Read the model definition and answer for the solid it produces. Units are mm, in the model's axes. Round coordinates to 2 decimals unless told otherwise and drop trailing zeros. Order: outer loops, then holes, each group sorted by start corner. A loop starts at its lowest first (then second) coordinate and runs counter-clockwise, first axis right, second up.
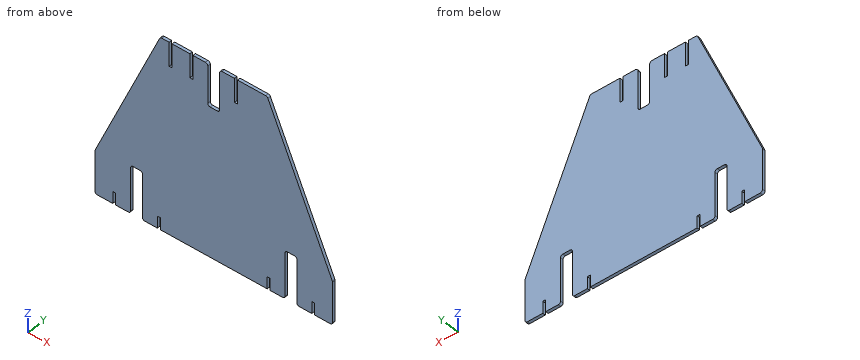
from build123d import *

# Parameters (mm, degrees)
BOSS_EXTRUDE1_DEPTH = 3.0988
FILLET1_R           = 2.54


with BuildPart() as part:
    # Sketch1 → Boss-Extrude1 (new body)
    with BuildSketch(Plane(origin=(0, 0, 0), x_dir=(1, 0, 0), z_dir=(0, 1, 0))):
        Polygon((6.35, -57.15), (-6.35, -57.15), (-6.35, -101.6), (-22.225, -101.6), (-22.225, -76.2), (-25.4, -76.2), (-25.4, -101.6), (-44.45, -101.6), (-44.45, -76.2), (-47.625, -76.2), (-47.625, -101.6), (-57.15, -101.6), (-127, 55.88), (-127, 101.6), (-107.95, 101.6), (-107.95, 88.9), (-104.775, 88.9), (-104.775, 101.6), (-88.9, 101.6), (-88.9, 50.8), (-76.2, 50.8), (-76.2, 101.6), (-60.325, 101.6), (-60.325, 88.9), (-57.15, 88.9), (-57.15, 101.6), (57.15, 101.6), (57.15, 88.9), (60.325, 88.9), (60.325, 101.6), (76.2, 101.6), (76.2, 50.8), (88.9, 50.8), (88.9, 101.6), (104.775, 101.6), (104.775, 88.9), (107.95, 88.9), (107.95, 101.6), (127, 101.6), (127, 55.88), (57.15, -101.6), (25.4, -101.6), (25.4, -76.2), (22.225, -76.2), (22.225, -101.6), (6.35, -101.6), align=None)
    extrude(amount=BOSS_EXTRUDE1_DEPTH)

    # Fillet1
    fillet1_edges = [part.edges().sort_by_distance(p)[0] for p in [
        (88.9, 1.5494, -50.8),
        (88.9, 1.5494, -101.6),
        (127, 1.5494, -101.6),
        (127, 1.5494, -55.88),
        (57.15, 1.5494, 101.6),
        (6.35, 1.5494, 101.6),
        (6.35, 1.5494, 57.15),
        (-6.35, 1.5494, 57.15),
        (-6.35, 1.5494, 101.6),
        (-57.15, 1.5494, 101.6),
        (-127, 1.5494, -55.88),
        (-127, 1.5494, -101.6),
        (-88.9, 1.5494, -101.6),
        (-88.9, 1.5494, -50.8),
        (-76.2, 1.5494, -50.8),
        (-76.2, 1.5494, -101.6),
        (76.2, 1.5494, -101.6),
        (76.2, 1.5494, -50.8),
    ]]
    fillet(fillet1_edges, radius=FILLET1_R)


solid = part.part
Q1. A cutting plane is placed at B-B, the plane x = 82. Give the vertices of the cut face in (y, z).
Outcome:
outline: (0, -50.8) - (3.1, -50.8) - (3.1, 45.57) - (0, 45.57) - close
Q2. A cutting plane is placed at A-A, the plane z = -71. Give the vertices of the cut face in (x, y).
Outcome:
outline: (-127, 0) - (-88.9, 0) - (-88.9, 3.1) - (-127, 3.1) - close; (-76.2, 0) - (76.2, 0) - (76.2, 3.1) - (-76.2, 3.1) - close; (88.9, 0) - (127, 0) - (127, 3.1) - (88.9, 3.1) - close
Q3. A cutting plane is placed at C-C, the plane z = 22. Give the vertices of the cut face in (x, y).
Outcome:
outline: (-92.46, 0) - (92.46, 0) - (92.46, 3.1) - (-92.46, 3.1) - close
Q4. Flat-ended cylindrical pins translate along their axes: pin 1 (1.5 mm diameter, centred on x = -24, y = 2, fed in from +Z); pin 2 (1.5 mm diameter, centred on x = -81.5, y = 1, fed in from -Z); pin 3 (0.9 mm diameter, centred on x = 58.5, y = 1, fed in from -Z); pin 4 (1.5 mm diameter, centred on x = -15, z = -65.5, fed in from -Y). Find the tip coordinate at first contact, or state that the pin passes through.
Outcome:
pin 1: stops at z = 76.2
pin 2: stops at z = -50.8
pin 3: stops at z = -88.9
pin 4: stops at y = 0
Q5. Straight lines are drawn through the part: probe 1 along X at (y, z) = (1, -67); probe 2 along X at (y, z) = (1.2, 70); probe 3 along Z at (x, y) = (-106, 1.4). For each, find the intervals that lie inside material, in ascending order.
Outcome:
probe 1: x = -127 to -88.9, -76.2 to 76.2, 88.9 to 127
probe 2: x = -71.17 to -6.35, 6.35 to 71.17
probe 3: z = -88.9 to -8.53
